Model file for the job. Use its own axes, mm. Face numbers are marked on the shaded views. A direction names the side the tool comes from. Round coordinates to 2 decimals unless told otherwise and drop trailing zeros. Loops run counter-clockwise (first coordinate to the right, second up) from the corner with the lowest first, then second, coordinate; pieces in that order, holes last. Notation, with made-up numbers: (13, 74) - (42, 74) arc R25 ccw to (42, 111) - close; hole circle Ø10 at (50, 28). An arc over 180 degrees is marked (long way). Use one line per item in the form item = value.
from build123d import *

# Parameters (mm, degrees)
SKETCH1_R               = 13.5
SKETCH1_R_2             = 10
BOSS_EXTRUDE1_DEPTH     = 30
BOSS_EXTRUDE2_START     = 30
SKETCH1_3_R             = 16
SKETCH1_3_R_2           = 13.5
SKETCH1_3_R_3           = 10
BOSS_EXTRUDE2_DEPTH     = 4
SKETCH2_R               = 7.5
BOSS_EXTRUDE3_DEPTH     = 2
CUT_EXTRUDE1_REACH      = 68.94
CUT_EXTRUDE1_END_RADIUS = 13.5
SKETCH2_3_R             = 2.5
CUT_EXTRUDE2_DEPTH      = 67.940271885
CUT_EXTRUDE2_DEPTH_BACK = 67.940271885
SKETCH3_R               = 2.5


with BuildPart() as part:
    # Sketch1 → Boss-Extrude1 (new body)
    with BuildSketch(Plane(origin=(0, 0, 0), x_dir=(1, 0, 0), z_dir=(0, 1, 0))):
        with Locations(Location((0, 0, 0), (0, 0, 270))):
            Circle(SKETCH1_R)
        with Locations(Location((0, 0, 0), (0, 0, 270))):
            Circle(SKETCH1_R_2, mode=Mode.SUBTRACT)
    extrude(amount=BOSS_EXTRUDE1_DEPTH)

    # Sketch1<3> → Boss-Extrude2 (add)
    # profile 1 of 3: a face of its own
    with BuildSketch(Plane(origin=(0, 0, 0), x_dir=(1, 0, 0), z_dir=(0, 1, 0)).offset(BOSS_EXTRUDE2_START)):
        with Locations(Location((0, 0, 0), (0, 0, 270))):
            Circle(SKETCH1_3_R)
        with Locations(Location((0, 0, 0), (0, 0, 270))):
            Circle(SKETCH1_3_R_2, mode=Mode.SUBTRACT)
    # profile 2 of 3: a face of its own
    with BuildSketch(Plane(origin=(0, 0, 0), x_dir=(1, 0, 0), z_dir=(0, 1, 0)).offset(BOSS_EXTRUDE2_START)):
        with Locations(Location((0, 0, 0), (0, 0, 270))):
            Circle(SKETCH1_3_R_2)
        with Locations(Location((0, 0, 0), (0, 0, 270))):
            Circle(SKETCH1_3_R_3, mode=Mode.SUBTRACT)
    # profile 3 of 3: a face of its own
    with BuildSketch(Plane(origin=(0, 0, 0), x_dir=(1, 0, 0), z_dir=(0, 1, 0)).offset(BOSS_EXTRUDE2_START)):
        with Locations(Location((0, 0, 0), (0, 0, 270))):
            Circle(SKETCH1_3_R_3)
    extrude(amount=BOSS_EXTRUDE2_DEPTH)

    # Sketch2 → Boss-Extrude3 (add, symmetric)
    with BuildSketch(Plane(origin=(0, 0, 0), x_dir=(0, 0, -1), z_dir=(1, 0, 0))):
        with BuildLine():
            Line((13, 50), (13, 34))
            Line((13, 34), (-13, 34))
            Line((-13, 34), (-13, 50))
            ThreePointArc((-13, 50), (0, 63), (13, 50))
        make_face()
        with Locations((0, 50)):
            Circle(SKETCH2_R, mode=Mode.SUBTRACT)
    extrude(amount=BOSS_EXTRUDE3_DEPTH, both=True)

    # Cut-Extrude1: up to this cylinder (the profile starts inside it)
    cut_extrude1_end = Plane(origin=(0, 18, 0), z_dir=(0, -1, 0)) * Cylinder(CUT_EXTRUDE1_END_RADIUS, 165.88, mode=Mode.PRIVATE)
    # Sketch2<3> → Cut-Extrude1 (cut, up to the surface)
    with BuildSketch(Plane(origin=(0, 0, 0), x_dir=(0, 0, -1), z_dir=(1, 0, 0)), mode=Mode.PRIVATE) as cut_extrude1_sk1:
        with Locations(Location((0, 18, 0), (0, 0, 180))):
            Circle(SKETCH2_3_R)
    cut_extrude1_tool1 = extrude(cut_extrude1_sk1.sketch, amount=CUT_EXTRUDE1_REACH, mode=Mode.PRIVATE) & cut_extrude1_end
    add(cut_extrude1_tool1.solids().sort_by_distance((0, 18, 0))[0], mode=Mode.SUBTRACT)

    # Sketch3 → Cut-Extrude2 (cut, two sides: drawn at the far end of the back side and taken through both)
    with BuildSketch(Plane.XY.offset(-CUT_EXTRUDE2_DEPTH_BACK)):
        with Locations((0, 10)):
            Circle(SKETCH3_R)
    extrude(amount=CUT_EXTRUDE2_DEPTH + CUT_EXTRUDE2_DEPTH_BACK, mode=Mode.SUBTRACT)


solid = part.part
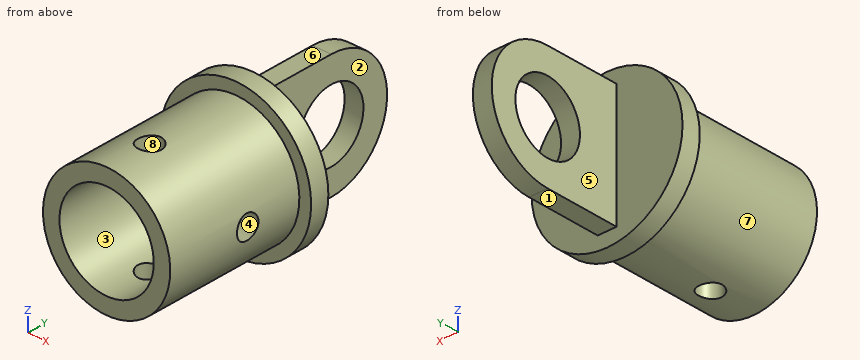
1. Pull direction X, two halves, no side cores. Call the marked faces 6, 7 and 8: +X half, -X half, draft (parallel to the pull), parting line (faces both ways), or undercut.
Geometry check:
face_6 = draft
face_7 = parting line
face_8 = undercut
2. Cut at C-C, the plane z = 6.5. Give the cut face in (x, y), plus the area to 3 significant figures.
Geometry check:
outline = (-14.62, 30) - (-11.83, 30) - (-11.83, 0) - (-7.6, 0) - (-7.6, 30) - (7.6, 30) - (7.6, 0) - (11.83, 0) - (11.83, 30) - (14.62, 30) - (14.62, 34) - (2, 34) - (2, 46.26) - (-2, 46.26) - (-2, 34) - (-14.62, 34) - close; (-2, 53.74) - (2, 53.74) - (2, 61.26) - (-2, 61.26) - close
area = 450 mm^2
3. Cut at B-B, the plane z = 0. Give the cut face in (x, y).
Geometry check:
outline = (-16, 30) - (-13.5, 30) - (-13.5, 0) - (-10, 0) - (-10, 30) - (10, 30) - (10, 20.5) - (13.5, 20.5) - (13.5, 30) - (16, 30) - (16, 34) - (2, 34) - (2, 42.5) - (-2, 42.5) - (-2, 34) - (-16, 34) - close; (-2, 57.5) - (2, 57.5) - (2, 63) - (-2, 63) - close; (10, 0) - (13.5, 0) - (13.5, 15.5) - (10, 15.5) - close
4. Wall check: probe 1 along X at (y, z) = (55, -8); probe 2 along Y at (x, z) = (-3, 3); probe 3 along Y at (x, z) = (0.5, -4). Give the ranges that are in metal, low to high.
Geometry check:
probe_1 = -2 to 2
probe_2 = 30 to 34
probe_3 = 30 to 43.66, 56.34 to 62.37
5. Cut at A-A, the plane x = 0. Give the cut face in (y, z), plus the area to 3 significant figures.
Geometry check:
outline = (0, -13.5) - (7.5, -13.5) - (7.5, -10) - (0, -10) - close; (0, 10) - (7.5, 10) - (7.5, 13.5) - (0, 13.5) - close; (12.5, -13.5) - (30, -13.5) - (30, -16) - (34, -16) - (34, -13) - (50, -13) arc R13 ccw to (50, 13) - (34, 13) - (34, 16) - (30, 16) - (30, 13.5) - (12.5, 13.5) - (12.5, 10) - (30, 10) - (30, -10) - (12.5, -10) - close; hole circle Ø15 at (50, 0)
area = 808 mm^2
6. Cut at D-D, the plane y = 10. Give the cut face in (x, z), plus the area to 3 significant figures.
Geometry check:
outline = (-2.5, -13.27) - (-2.5, -9.68) arc R10 cw to (-2.5, 9.68) - (-2.5, 13.27) arc R13.5 ccw to start; (2.5, -13.27) arc R13.5 ccw to (2.5, 13.27) - (2.5, 9.68) arc R10 cw to (2.5, -9.68) - close
area = 223 mm^2
7. Tool access for the marked faces 1, 2, 3, 4 and 5: list every direction of +Z, -Z, +X, -X, +Y, -Y with a clear straight run to the whole face (end or side of a thin tool).
Geometry check:
face_1 = -Z, +X, -X, +Y
face_2 = +Z, -Z, +X, +Y
face_3 = -Y
face_4 = +X
face_5 = +Z, -Z, -X, +Y
8. Flat gauge pins, fed straight in: pin 1 (8 mm diameter, centred on x = -4.5, y = 40, fed in from -Z); pin 2 (6 mm diameter, centred on y = 14.5, z = -4, fed in from +X); pin 3 (6 mm diameter, centred on x = 0, y = 10, fed in from -Z); pin 4 (4 mm diameter, centred on x = 0, y = 10, fed in from -Z). Where does each tip first touch, or does it go through?
Geometry check:
pin_1 = -13
pin_2 = 13.46
pin_3 = -13.5
pin_4 = through
